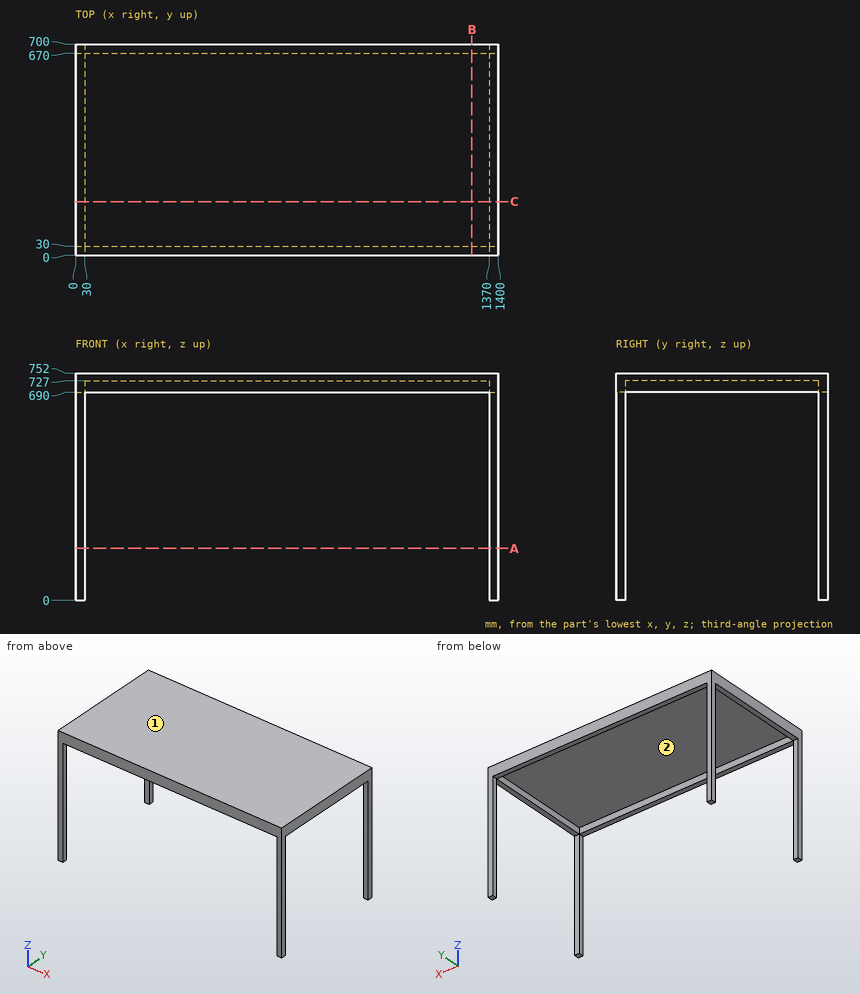
Verification items for this drawing (mm, ordinates from the low corner). A direction names the side the tool comes from. Round coordinates to 2 decimals unless told otherwise and drop trailing zeros. Order: outer loops, then holes, each group sorted by start corner. A loop starts at its lowest first (then second) coordinate and runs counter-clockwise, first axis right, second up. Notation, with made-up numbers: M -18,13 L 12,13 A24 cw 12,38 Z; hole C -29.75,-14 d8. An arc over 180 degrees is marked long. Answer in a Markdown table with one row per item. Add a question column.
Item 1: Sectioned sample at B-B, the plane x = 1312.5. Enter the section's corners in (y, z).
Item 2: Set-up check for the marked faces 1 and 2: record each of +Z, -Z, +X, -X, +Y, -Y from which the full face is reachable in a straight line by a thin tool's end or side.
Item 3: Sectioned sample at C-C, the plane y = 177.5. Enter the section's corners in (x, z), plus the area to 3 significant figures.
Item 4: Depth check by flat-ended pin: pin 1 Ø15 at (x, y) = (396, 12) entering from -Z; pin 2 Ø1.5 at (x, y) = (897.5, 153) entering from -Z. Enter the tip coordinate at first touch or a pass-through.
Item 5: Material ranges on L1, parallel to X at y = 671, z = 367; L2, parallel to Z at x = 768, y = 66, recorded low to high. Write a range as [from, to].
Item 6: Sectioned sample at A-A, the plane z = 172. Enter the section's corners in (x, y), plus the area to 3 significant figures.
Filled in:
| question | item | result |
|---|---|---|
| 1 | outline | M 0,690 L 30,690 L 30,727 L 670,727 L 670,690 L 700,690 L 700,752 L 0,752 Z |
| 2 | face 1 | +Z, +X, -X, +Y, -Y |
| 2 | face 2 | -Z |
| 3 | outline | M 0,690 L 30,690 L 30,727 L 1370,727 L 1370,690 L 1400,690 L 1400,752 L 0,752 Z |
| 3 | area | 37,200 mm² |
| 4 | pin 1 | stops at z = 690 |
| 4 | pin 2 | stops at z = 727 |
| 5 | L1 | x = [0, 30], [1370, 1400] |
| 5 | L2 | z = [727, 752] |
| 6 | outline | M 0,0 L 30,0 L 30,30 L 0,30 Z; M 0,670 L 30,670 L 30,700 L 0,700 Z; M 1370,0 L 1400,0 L 1400,30 L 1370,30 Z; M 1370,670 L 1400,670 L 1400,700 L 1370,700 Z |
| 6 | area | 3,600 mm² |
